The listing builds one solid part. Answer for the finished solid, in the listing's coordinates (mm). A direction names the side the tool comes from. Give positions to 0.01 mm unless a question says otherwise; leave off trailing zeros. Order: outer loops, then holes, each group sorted by start corner. A loop starts at its lowest first (then second) coordinate and runs counter-clockwise, first axis right, second up.
```python
from build123d import *

# Parameters (mm, degrees)
SKETCH1_R           = 3.575
BOSS_EXTRUDE1_DEPTH = 20
FILLET1_R           = 5
SKETCH5_W           = 24
SKETCH5_H           = 7
CUT_EXTRUDE1_DEPTH  = 7
SKETCH6_R           = 1.7
CUT_EXTRUDE2_DEPTH  = 8
SKETCH3_R           = 3.7
CUT_EXTRUDE3_DEPTH  = 0.85


with BuildPart() as part:
    # Sketch1 → Boss-Extrude1 (new body)
    with BuildSketch(Plane.XY):
        with BuildLine():
            Line((-200, 25), (-30, 0))
            Line((-30, 0), (0, 0))
            Line((0, 0), (0, 26.5))
            ThreePointArc((0, 26.5), (-2.872281323, 28.633974596), (-1.658312395, 32))
            Line((-1.658312395, 32), (0, 32))
            Line((0, 32), (0, 32.5))
            Line((0, 32.5), (0, 50))
            Line((0, 50), (-200, 50))
            Line((-200, 50), (-200, 25))
        make_face()
        with Locations((-190, 37.5)):
            Circle(SKETCH1_R, mode=Mode.SUBTRACT)
    extrude(amount=BOSS_EXTRUDE1_DEPTH)

    # Fillet1
    fillet1_edges = [part.edges().sort_by_distance(p)[0] for p in [
        (-200, 25, 10),
        (-200, 50, 10),
    ]]
    fillet(fillet1_edges, radius=FILLET1_R)

    # Sketch5 → Cut-Extrude1 (cut)
    with BuildSketch(Plane(origin=(0, 50, 0), x_dir=(1, 0, 0), z_dir=(0, 1, 0))):
        with Locations((-20, -10)):
            Rectangle(SKETCH5_W, SKETCH5_H)
    cut_extrude1 = extrude(amount=-CUT_EXTRUDE1_DEPTH, mode=Mode.SUBTRACT)

    # Sketch6 → Cut-Extrude2 (cut)
    with BuildSketch(Plane.ZY.offset(8)):
        with Locations((10, 46.5)):
            Circle(SKETCH6_R)
    cut_extrude2 = extrude(amount=-CUT_EXTRUDE2_DEPTH, mode=Mode.SUBTRACT)

    # Mirror1: Cut-Extrude1, Cut-Extrude2 across plane
    add(cut_extrude1.mirror(Plane.ZX.offset(25)), mode=Mode.SUBTRACT)
    add(cut_extrude2.mirror(Plane.ZX.offset(25)), mode=Mode.SUBTRACT)

    # Sketch3 → Cut-Extrude3 (cut)
    with BuildSketch(Plane.XY.offset(20)):
        with Locations((-190, 37.5)):
            Circle(SKETCH3_R)
    cut_extrude3 = extrude(amount=-CUT_EXTRUDE3_DEPTH, mode=Mode.SUBTRACT)

    # Mirror2: Cut-Extrude3 across plane
    add(cut_extrude3.mirror(Plane.XY.offset(10)), mode=Mode.SUBTRACT)


solid = part.part
```
1) For a pull along X with two mould halves and no side action, classify faces 4 (the cylindrical face through (-2.856, 28.583, 9.86)), 5 (the flat face through (-79, 31, 0)), 6 (the flat face through (-20, 47, 6.5)) as +X half, -X half, draft (parallel to the pull), parting line (faces both ways), or undercut.
Geometry says:
face 4: +X half
face 5: draft
face 6: undercut
2) Straight lines are drawn through the part: probe 1 along Z at (x, y) = (-1.75, 3.5); probe 2 along Y at (x, z) = (-190, 19.7); probe 3 along Z at (x, y) = (-3, 46). For each, find the intervals that lie inside material, in ascending order.
Geometry says:
probe 1: z = 0 to 8.3, 11.7 to 20
probe 2: y = 23.53 to 33.8, 41.2 to 50
probe 3: z = 0 to 8.38, 11.62 to 20
3) Find section D-D (y = 15). Write down the section's boundary in (x, z).
Geometry says:
outline: (-132, 0) - (0, 0) - (0, 20) - (-132, 20) - close
4) Find section B-B (y = 3.5). Write down the section's boundary in (x, z), then the cut area to 3 significant figures.
Geometry says:
outline: (-53.8, 0) - (0, 0) - (0, 8.3) - (-8, 8.3) - (-8, 6.5) - (-32, 6.5) - (-32, 13.5) - (-8, 13.5) - (-8, 11.7) - (0, 11.7) - (0, 20) - (-53.8, 20) - close
area: 881 mm2
5) Find section A-A (x = -190). Write down the section's boundary in (y, z) (3 decimals).
Geometry says:
outline: (23.529, 0) - (33.8, 0) - (33.8, 0.85) - (33.925, 0.85) - (33.925, 19.15) - (33.8, 19.15) - (33.8, 20) - (23.529, 20) - close; (41.075, 0.85) - (41.2, 0.85) - (41.2, 0) - (50, 0) - (50, 20) - (41.2, 20) - (41.2, 19.15) - (41.075, 19.15) - close
6) A tool of negligible diameter and unlimited length cuts with its end or side. For faces 1 (the flat face through (-20, 47, 13.5)), 2 (the cylindrical face through (-186.47, 38.61, 0.42)), 3 (the flat face through (-20, 7, 10)), from which of +Z, -Z, +X, -X, +Y, -Y can it reach the whole face along a straight path? Write none if from no direction.
Geometry says:
face 1: +Y
face 2: -Z
face 3: -Y
7) Find section C-C (x = -60). Write down the section's boundary in (y, z), then the cut area to 3 significant figures.
Geometry says:
outline: (4.41, 0) - (50, 0) - (50, 20) - (4.41, 20) - close
area: 912 mm2
